Geometry check sheet. Reference: the model listing, model coordinates, mm. Face numbers are marked on the shaded views. A direction names the side the tool comes from. Give positions to 0.01 mm unless a question says otherwise; leave off trailing zeros. Order: outer loops, then holes, each group sorted by start corner. A loop starts at its lowest first (then second) coordinate and runs counter-clockwise, first axis right, second up. Notation, with made-up numbers: M -8.75,17 L 47.25,17 A10 ccw 47.25,35 Z; hole C 71.25,40.5 d7. An arc over 180 degrees is marked long. Put each result on its own line as item: value. Start each with the question number.
Q1. Go/stop test with flat-tipped pins: pin 1 (0.6 mm diameter, centred on x = -10, z = 0, fed in from +Y); pin 2 (1.5 mm diameter, centred on x = 12.5, y = 8, fed in from +Z); pin 3 (10.5 mm diameter, centred on x = -4.5, z = 3.5, fed in from +Y); pin 4 (2.5 mm diameter, centred on x = 6.5, z = -4.5, fed in from -Y). Record where each tip stops, or that it passes through.
Q2. Section check D-D on z = 0. Record the cut outline in (x, y).
Q3. Section check B-B on z = 7.75. Record the cut outline in (x, y), then the cut area to 3 significant figures.
Q4. Access from +Z, -Z, +X, -X, +Y, -Y to the whole of each face (thin tool, end or side, straight path). Record for the marked faces 4, 5 and 6.
Q5. Mould release check, pull along Z, two halves, no side actions. Record for the marked faces 1, 2 and 3: +Z half, -Z half, draft (parallel to the pull), parting line (faces both ways), or undercut.
Q6. Section check A-A on x = 6.5. Record the cut outline in (y, z).
Q7. Section check C-C on y = 5. Record the cut outline in (x, z), then the cut area to 3 significant figures.
Q8. Material ranges on L1, parallel to X at y = 3.45, z = 0; L2, parallel to Z at x = 11, y = 5.5; L3, parallel to Z at x = 1, y = 4.5, recorded low to high.
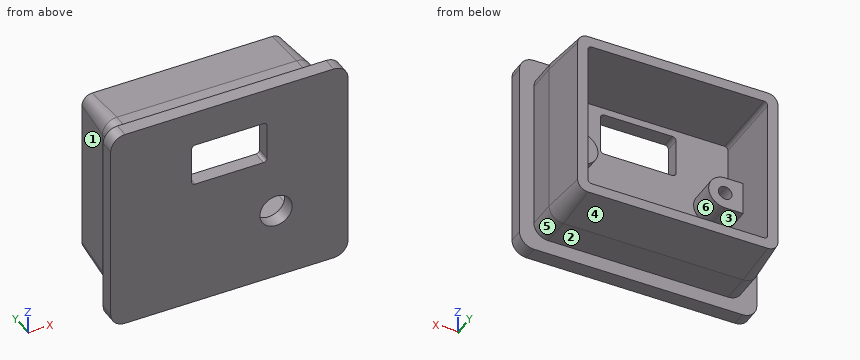
```python
from build123d import *
from OCP.BRepFilletAPI import BRepFilletAPI_MakeChamfer

# Parameters (mm, degrees)
SKETCH1_W           = 33
SKETCH1_H           = 29
BOSS_EXTRUDE1_DEPTH = 2
SKETCH2_W           = 29
SKETCH2_H           = 25
SKETCH2_W_2         = 25
SKETCH2_H_2         = 21
BOSS_EXTRUDE2_DEPTH = 10.5
SKETCH3_W           = 10.5
SKETCH3_H           = 6
CUT_EXTRUDE1_DEPTH  = 2
SKETCH4_R           = 2.25
CUT_EXTRUDE2_DEPTH  = 2
SKETCH5_R           = 0.95
BOSS_EXTRUDE3_DEPTH = 4
FILLET1_R           = 2
FILLET2_R           = 0.5
CHAMFER1_SIZE       = 6.5
CHAMFER1_SIZE2      = 0.568676313


with BuildPart() as part:
    # Sketch1 → Boss-Extrude1 (new body)
    with BuildSketch(Plane(origin=(0, 0, 0), x_dir=(1, 0, 0), z_dir=(0, 1, 0))):
        Rectangle(SKETCH1_W, SKETCH1_H)
    extrude(amount=BOSS_EXTRUDE1_DEPTH)

    # Sketch2 → Boss-Extrude2 (add)
    with BuildSketch(Plane(origin=(0, 2, 0), x_dir=(1, 0, 0), z_dir=(0, 1, 0))):
        Rectangle(SKETCH2_W, SKETCH2_H)
        Rectangle(SKETCH2_W_2, SKETCH2_H_2, mode=Mode.SUBTRACT)
    extrude(amount=BOSS_EXTRUDE2_DEPTH)

    # Sketch3 → Cut-Extrude1 (cut)
    with BuildSketch(Plane(origin=(0, 2, 0), x_dir=(1, 0, 0), z_dir=(0, 1, 0))):
        with Locations((0, -6.5)):
            Rectangle(SKETCH3_W, SKETCH3_H)
    extrude(amount=-CUT_EXTRUDE1_DEPTH, mode=Mode.SUBTRACT)

    # Sketch4 → Cut-Extrude2 (cut)
    with BuildSketch(Plane(origin=(0, 2, 0), x_dir=(1, 0, 0), z_dir=(0, 1, 0))):
        with Locations(Location((6.5, 4.5, 0), (0, 0, 270))):
            Circle(SKETCH4_R)
    extrude(amount=-CUT_EXTRUDE2_DEPTH, mode=Mode.SUBTRACT)

    # Sketch5 → Boss-Extrude3 (add)
    with BuildSketch(Plane(origin=(0, 2, 0), x_dir=(1, 0, 0), z_dir=(0, 1, 0))):
        with BuildLine():
            Line((-10, 2.3), (-12.5, 2.3))
            Line((-12.5, 2.3), (-12.5, -2.3))
            Line((-12.5, -2.3), (-10, -2.3))
            ThreePointArc((-10, -2.3), (-7.7, 0), (-10, 2.3))
        make_face()
        with Locations(Location((-10, 0, 0), (0, 0, 270))):
            Circle(SKETCH5_R, mode=Mode.SUBTRACT)
    boss_extrude3 = extrude(amount=BOSS_EXTRUDE3_DEPTH)

    # Mirror1: Boss-Extrude3 across plane
    add(boss_extrude3.mirror(Plane(origin=(0, 0, 0), x_dir=(0, 0, 1), z_dir=(1, 0, 0))))

    # Fillet1
    fillet1_edges = [part.edges().sort_by_distance(p)[0] for p in [
        (14.5, 7.25, 12.5),
        (14.5, 7.25, -12.5),
        (-14.5, 7.25, -12.5),
        (-14.5, 7.25, 12.5),
        (16.5, 1, 14.5),
        (-16.5, 1, 14.5),
        (-16.5, 1, -14.5),
        (16.5, 1, -14.5),
    ]]
    fillet(fillet1_edges, radius=FILLET1_R)

    # Fillet2
    fillet2_edges = [part.edges().sort_by_distance(p)[0] for p in [
        (12.5, 7.25, -10.5),
        (-12.5, 7.25, -10.5),
        (-12.5, 7.25, 10.5),
        (12.5, 7.25, 10.5),
        (-5.25, 1, 3.5),
        (-5.25, 1, 9.5),
        (5.25, 1, 9.5),
        (5.25, 1, 3.5),
    ]]
    fillet(fillet2_edges, radius=FILLET2_R)

    # Chamfer1: one chamfer whose edges measure the first distance from different faces: ONE call of the kernel's chamfer builder (chamfer() names one face for all edges)
    chamfer1_edges_1 = [part.edges().sort_by_distance(p)[0] for p in [
        (-14.5, 12.5, 0),
    ]]
    chamfer1_side_1 = [part.faces().sort_by_distance(p)[0] for p in [
        (-14.5, 7.25, 0),
    ]]
    chamfer1_edges_2 = [part.edges().sort_by_distance(p)[0] for p in [
        (0, 12.5, -12.5),
    ]]
    chamfer1_side_2 = [part.faces().sort_by_distance(p)[0] for p in [
        (0, 7.25, -12.5),
    ]]
    chamfer1_edges_3 = [part.edges().sort_by_distance(p)[0] for p in [
        (14.5, 12.5, 0),
    ]]
    chamfer1_side_3 = [part.faces().sort_by_distance(p)[0] for p in [
        (14.5, 7.25, 0),
    ]]
    chamfer1_edges_4 = [part.edges().sort_by_distance(p)[0] for p in [
        (0, 12.5, 12.5),
    ]]
    chamfer1_side_4 = [part.faces().sort_by_distance(p)[0] for p in [
        (0, 7.25, 12.5),
    ]]
    chamfer1_edges_5 = [part.edges().sort_by_distance(p)[0] for p in [
        (13.914213562, 12.5, -11.914213562),
    ]]
    chamfer1_side_5 = [part.faces().sort_by_distance(p)[0] for p in [
        (13.914213562, 7.25, -11.914213562),
    ]]
    chamfer1_edges_6 = [part.edges().sort_by_distance(p)[0] for p in [
        (13.914213562, 12.5, 11.914213562),
    ]]
    chamfer1_side_6 = [part.faces().sort_by_distance(p)[0] for p in [
        (13.914213562, 7.25, 11.914213562),
    ]]
    chamfer1_edges_7 = [part.edges().sort_by_distance(p)[0] for p in [
        (-13.914213562, 12.5, 11.914213562),
    ]]
    chamfer1_side_7 = [part.faces().sort_by_distance(p)[0] for p in [
        (-13.914213562, 7.25, 11.914213562),
    ]]
    chamfer1_edges_8 = [part.edges().sort_by_distance(p)[0] for p in [
        (-13.914213562, 12.5, -11.914213562),
    ]]
    chamfer1_side_8 = [part.faces().sort_by_distance(p)[0] for p in [
        (-13.914213562, 7.25, -11.914213562),
    ]]
    chamfer1 = BRepFilletAPI_MakeChamfer(part.part.solid().wrapped)
    for e in chamfer1_edges_1:
        chamfer1.Add(CHAMFER1_SIZE, CHAMFER1_SIZE2, e.wrapped, chamfer1_side_1[0].wrapped)  # the first distance lies on this face
    for e in chamfer1_edges_2:
        chamfer1.Add(CHAMFER1_SIZE, CHAMFER1_SIZE2, e.wrapped, chamfer1_side_2[0].wrapped)  # the first distance lies on this face
    for e in chamfer1_edges_3:
        chamfer1.Add(CHAMFER1_SIZE, CHAMFER1_SIZE2, e.wrapped, chamfer1_side_3[0].wrapped)  # the first distance lies on this face
    for e in chamfer1_edges_4:
        chamfer1.Add(CHAMFER1_SIZE, CHAMFER1_SIZE2, e.wrapped, chamfer1_side_4[0].wrapped)  # the first distance lies on this face
    for e in chamfer1_edges_5:
        chamfer1.Add(CHAMFER1_SIZE, CHAMFER1_SIZE2, e.wrapped, chamfer1_side_5[0].wrapped)  # the first distance lies on this face
    for e in chamfer1_edges_6:
        chamfer1.Add(CHAMFER1_SIZE, CHAMFER1_SIZE2, e.wrapped, chamfer1_side_6[0].wrapped)  # the first distance lies on this face
    for e in chamfer1_edges_7:
        chamfer1.Add(CHAMFER1_SIZE, CHAMFER1_SIZE2, e.wrapped, chamfer1_side_7[0].wrapped)  # the first distance lies on this face
    for e in chamfer1_edges_8:
        chamfer1.Add(CHAMFER1_SIZE, CHAMFER1_SIZE2, e.wrapped, chamfer1_side_8[0].wrapped)  # the first distance lies on this face
    add(Compound.cast(chamfer1.Shape()), mode=Mode.REPLACE)


solid = part.part
```
Results found:
1. pin 1: stops at y = 2
1. pin 2: stops at z = 12.39
1. pin 3: stops at y = 6
1. pin 4: passes through
2. outline: M -16.5,0 L 16.5,0 L 16.5,2 L 14.5,2 L 14.5,6 L 13.93,12.5 L 12.5,12.5 L 12.5,6 L 10.95,6 L 10.95,2 L 9.05,2 L 9.05,6 L 7.7,6 L 7.7,2 L -7.7,2 L -7.7,6 L -9.05,6 L -9.05,2 L -10.95,2 L -10.95,6 L -12.5,6 L -12.5,12.5 L -13.93,12.5 L -14.5,6 L -14.5,2 L -16.5,2 Z
3. outline: M -16.5,0 L -5.25,0 L -5.25,2 L -12.5,2 L -12.5,12.5 L -13.93,12.5 L -14.5,6 L -14.5,2 L -16.5,2 Z; M 5.25,0 L 16.5,0 L 16.5,2 L 14.5,2 L 14.5,6 L 13.93,12.5 L 12.5,12.5 L 12.5,2 L 5.25,2 Z
3. area: 83.3 mm^2
4. face 4: -Z, +X, -X, +Y
4. face 5: -Z, +X, +Y
4. face 6: +Y
5. face 1: draft
5. face 2: -Z half
5. face 3: undercut
6. outline: M 0,-14.5 L 2,-14.5 L 2,-12.5 L 6,-12.5 L 12.5,-11.93 L 12.5,-10.5 L 2,-10.5 L 2,-6.75 L 0,-6.75 Z; M 0,-2.25 L 2,-2.25 L 2,10.5 L 12.5,10.5 L 12.5,11.93 L 6,12.5 L 2,12.5 L 2,14.5 L 0,14.5 Z
7. outline: M -14.5,-10.5 A2 ccw -12.5,-12.5 L 12.5,-12.5 A2 ccw 14.5,-10.5 L 14.5,10.5 A2 ccw 12.5,12.5 L -12.5,12.5 A2 ccw -14.5,10.5 Z; hole M -12.5,-10 A0.5 ccw -12,-10.5 L 12,-10.5 A0.5 ccw 12.5,-10 L 12.5,-2.3 L 10,-2.3 A2.3 cw 10,2.3 L 12.5,2.3 L 12.5,10 A0.5 ccw 12,10.5 L -12,10.5 A0.5 ccw -12.5,10 L -12.5,2.3 L -10,2.3 A2.3 cw -10,-2.3 L -12.5,-2.3 Z; hole C -10,0 d1.9; hole C 10,0 d1.9
7. area: 231 mm^2
8. L1: x = -14.5 to -10.95, -9.05 to -7.7, 7.7 to 9.05, 10.95 to 14.5
8. L2: z = -12.5 to -10.5, -2.3 to 2.3, 10.5 to 12.5
8. L3: z = -12.5 to -10.5, 10.5 to 12.5
